Part model, mm, in its own coordinate system. Round coordinates to 2 decimals unless told otherwise and drop trailing zeros. Loops run counter-clockwise (first coordinate to the right, second up) from the corner with the lowest first, then second, coordinate; pieces in that order, holes last. Notation, with made-up numbers: (-23.5, -17.5) -> (-7.5, -17.5) arc R11 cw to (-7.5, -7.5) -> close; hole circle Ø7 at (38, 41.25). An arc over 180 degrees is marked (long way). Answer as CSV lines item,"result".
Autodesk Inventor part; units mm, degrees
ref_plane "YZ Plane" through (0, 0, 0) normal (1, 0, 0) x (0, 1, 0)
ref_plane "XZ Plane" through (0, 0, 0) normal (0, 1, 0) x (-1, 0, 0)
ref_plane "XY Plane" through (0, 0, 0) normal (0, 0, 1) x (1, 0, 0)
sketch "Sketch1" plane through (0, 0, 0) normal (0, 0, 1) x (1, 0, 0)
  line L0 (-750, 0) -> (750, 0) construction
  line L1 (750, 0) -> (750, -2100) construction
  line L2 (750, -2100) -> (110, -2700) construction
  line L3 (108.907697, -2700) -> (-108.907697, -2700) construction
  line L4 (-110, -2700) -> (-750, -2100) construction
  line L5 (-750, -2100) -> (-750, 0) construction
  arc A0 (745.236855, 0.447083) -> (-745.236855, 0.447083) centre (0, -7964.766161) ccw construction
  arc A1 (-750.626493, -4.742884) -> (-777.58325, -235) centre (7180.794412, -1050) ccw construction
  arc A2 (-777.58325, -235) -> (-750.128547, -2099.028611) centre (7180.794412, -1050) ccw construction
  arc A3 (750.128547, -2099.028611) -> (777.58325, -235) centre (-7180.794412, -1050) ccw
  arc A4 (777.58325, -235) -> (750.626493, -4.742884) centre (-7180.794412, -1050) ccw construction
  line L6 (-777.58325, -235) -> (777.58325, -235) construction
  arc A5 (-749.322934, -2100.70831) -> (-677.569881, -2174.801078) centre (5033.298449, 3427.518345) ccw construction
  line L7 (-750, -2100) -> (750, -2100) construction
  line L8 (-547.172872, -2035.710935) -> (-801.083389, -2306.54882) construction
  arc A6 (-677.569881, -2174.801078) -> (-110.836747, -2699.297556) centre (5033.298449, 3427.518345) ccw construction
  arc A7 (-745.236855, 0.447083) -> (-750.626493, -4.742884) centre (-744.677927, -5.526826) ccw construction
  arc A8 (750.626493, -4.742884) -> (745.236855, 0.447083) centre (744.677927, -5.526826) ccw construction
  arc A9 (-750.128547, -2099.028611) -> (-749.322934, -2100.70831) centre (-747.154451, -2098.635225) ccw construction
  arc A10 (110.836747, -2699.297556) -> (677.569881, -2174.801078) centre (-5033.298449, 3427.518345) ccw construction
  line L9 (553.81945, -2042.800618) -> (794.436811, -2299.459137) construction
  arc A11 (677.569881, -2174.801078) -> (749.322934, -2100.70831) centre (-5033.298449, 3427.518345) ccw
  arc A12 (749.322934, -2100.70831) -> (750.128547, -2099.028611) centre (747.154451, -2098.635225) ccw
  arc A13 (-110.836747, -2699.297556) -> (-108.907697, -2700) centre (-108.907697, -2697) ccw construction
  arc A14 (108.907697, -2700) -> (110.836747, -2699.297556) centre (108.907697, -2697) ccw construction
  point P0 (0, 0)
  point P1 (0, 0)
  point P2 (0, 0)
  point P3 (0, -2700)
  point P4 (-674.128131, -2171.129877)
  point P5 (674.128131, -2171.129877)
  dimension "d19" = 1500
  dimension "d20" = 2100
  dimension "d21" = 220
  dimension "d22" = 2700
  dimension "d23" = 8000
  dimension "d24" = 8000
  dimension "d25" = 8000
  dimension "d26" = 235
  dimension "d27" = 8000
  dimension "d28" = 104
  dimension "d29" = 6
  dimension "d30" = 3
  dimension "d31" = 8000
  dimension "d32" = 104
  dimension "d33" = 3
contour flange "Contour Flange1" sketch "Sketch1" thickness 3 bend radius 3 width 1000 along (0, 0, 1) mid plane no both sides no wall seen from (713.565816, -2137.870332, 0) lies toward (0.718358, -0.6956736, 0) curves A11 A12 A3
bend "Bend1"
corner "Corner1"
equation "\"d19\" = d34"
equation "\"d20\" = d35"
equation "\"d21\" = d36"
equation "\"d24\" = d38"
equation "\"d25\" = d38"
equation "\"d26\" = d39"
equation "\"d27\" = d38"
equation "\"d29\" = d41 + d42"
equation "\"d30\" = d41"
equation "\"d31\" = d38"
equation "\"d8\" = Thickness"
equation "\"d9\" = BendReliefWidth"
equation "\"d10\" = BendReliefDepth"
equation "\"d11\" = MinimumRemnant"
equation "\"d12\" = TransitionRadius"
equation "\"d14\" = BendRadius"
equation "\"d16\" = CornerReliefSize"
equation "\"d17\" = GapSize"
equation "\"d18\" = JacobiRadiusSize"
equation "\"BendRadius\" = Thickness"
equation "\"BendReliefWidth\" = Thickness"
equation "\"BendReliefDepth\" = 0.5 * Thickness"
equation "\"CornerReliefSize\" = 4 * Thickness"
equation "\"MinimumRemnant\" = 2 * Thickness"
equation "\"TransitionRadius\" = BendRadius"
equation "\"JacobiRadiusSize\" = BendRadius"
equation "\"GapSize\" = Thickness"
equation "\"d42\" = d41"
properties part number "МОО 020 лист борт 1  Глеб_CPY"
Q1. Drill centre lines: line 1 along X through (y, z) = (-578, 859.5); line 2 along Y through (x, z) = (728.5, 173); line 3 along Y through (x, z) = (687, 858.5). Where is each one in solid material? Low to high.
Geometry results:
line 1,"805.27 to 808.27"
line 2,"-2126.73 to -2122.41"
line 3,"-2169.46 to -2165.17"
Q2. Drop flat-ended pins along their axis: P1, Ø12, axis at x = 737, z = 373.5, coming from the +Y side; P2, Ø8, axis at x = 713, z = 216.5, coming from the +Y side; P3, Ø1, axis at x = 719, z = 425, coming from the +Y side. Give the stop position or say it passes through.
Geometry results:
P1,"y = -2107.31"
P2,"y = -2134.32"
P3,"y = -2131.74"
Q3. Saw through at A-A, the plane z = 534.5. Write the cut outline in (x, y), then the cut area to 3 significant figures.
Geometry results:
outline,"(677.57, -2174.8) -> (679.71, -2176.9) arc R8003.01 ccw to (751.49, -2102.78) arc R6 ccw to (753.1, -2099.42) arc R8003 ccw to (780.57, -234.69) -> (777.58, -235) arc R8000 cw to (750.13, -2099.03) arc R3 cw to (749.32, -2100.71) arc R8000.01 cw to start"
area,"5,920 mm2"
Q4. Saw through at B-B, the plane x = 716. Write the cut outline in (y, z), then the cut area to 3 significant figures.
Geometry results:
outline,"(-2139.67, 0) -> (-2135.36, 0) -> (-2135.36, 1000) -> (-2139.67, 1000) -> close"
area,"4,310 mm2"
Q5. Saw through at C-C, the plane y = -1016.5. Write the cut outline in (x, z), then the cut area to 3 significant figures.
Geometry results:
outline,"(819.14, 0) -> (822.14, 0) -> (822.14, 1000) -> (819.14, 1000) -> close"
area,"3,000 mm2"
